```python
from build123d import *

# Parameters (mm, degrees)
F0_R         = 1.6
F1_DEPTH     = 5
F2_DEPTH     = 1
F3_R         = 16
F3_R_2       = 14.5
F4_DEPTH     = 10
F5_SIZE2     = 1.5
F5_SIZE      = 1
F8_T4_ANGLE  = 185.4300536725
F8_S5_R      = 22.5
F8_T6_DEPTH  = 9
F8_T10_ANGLE = 185.4300536725
F8_S11_R     = 22.5
F8_T12_DEPTH = 9
F9_R         = 5
F10_DEPTH    = 3
F11_R        = 3.25
F12_DEPTH    = 5


# Not quite as in the source:
# - a fillet or chamfer that OpenCascade refuses, or shapes differently, is made with other operations: its cross-section is extruded or revolved along the edge and cut away or added
# - a feature of the source that left no trace in its solid (it failed there, or was rolled back) is left out


with BuildPart() as f1:
    # F0 (on Top) → F1 (new body)
    with BuildSketch(Plane.XY):
        with BuildLine():
            ThreePointArc((-22.1862745098, -3.7442253372), (-22.5, 0), (-22.1862745098, 3.7442253372))
            ThreePointArc((-22.1862745098, 3.7442253372), (-30.5, 0), (-22.1862745098, -3.7442253372))
        make_face()
        with Locations((-25.5, 0)):
            Circle(F0_R, mode=Mode.SUBTRACT)
        with BuildLine():
            ThreePointArc((-20.5, 0), (-20.9410183456, 2.0532136456), (-22.1862745098, 3.7442253372))
            ThreePointArc((-22.1862745098, 3.7442253372), (-22.5, 0), (-22.1862745098, -3.7442253372))
            ThreePointArc((-22.1862745098, -3.7442253372), (-20.9410183456, -2.0532136456), (-20.5, 0))
        make_face()
    extrude(amount=F1_DEPTH)



with BuildPart() as f1b:
    # F0 (on Top) → F1, piece 2 (new body)
    with BuildSketch(Plane.XY):
        with BuildLine():
            ThreePointArc((22.1862745098, 3.7442253372), (22.4214314493, 1.8786728733), (22.5, 0))
            ThreePointArc((22.5, 0), (22.4214314493, -1.8786728733), (22.1862745098, -3.7442253372))
            ThreePointArc((22.1862745098, -3.7442253372), (27.5532136456, -4.5589816544), (30.5, 0))
            ThreePointArc((30.5, 0), (27.5532136456, 4.5589816544), (22.1862745098, 3.7442253372))
        make_face()
        with Locations((25.5, 0)):
            Circle(F0_R, mode=Mode.SUBTRACT)
        with BuildLine():
            ThreePointArc((22.1862745098, -3.7442253372), (22.4214314493, -1.8786728733), (22.5, 0))
            ThreePointArc((22.5, 0), (22.4214314493, 1.8786728733), (22.1862745098, 3.7442253372))
            ThreePointArc((22.1862745098, 3.7442253372), (20.5, 0), (22.1862745098, -3.7442253372))
        make_face()
    extrude(amount=F1_DEPTH)


with BuildPart() as f1_1:
    add(f1.part)

    add(f1b.part)  # F2 merges F1b
    # F0 (on Top) → F2 (join)
    with BuildSketch(Plane.XY):
        with BuildLine():
            ThreePointArc((22.1862745098, -3.7442253372), (20.5, 0), (22.1862745098, 3.7442253372))
            ThreePointArc((22.1862745098, 3.7442253372), (0, 22.5), (-22.1862745098, 3.7442253372))
            ThreePointArc((-22.1862745098, 3.7442253372), (-20.9410183456, 2.0532136456), (-20.5, 0))
            ThreePointArc((-20.5, 0), (-20.9410183456, -2.0532136456), (-22.1862745098, -3.7442253372))
            ThreePointArc((-22.1862745098, -3.7442253372), (0, -22.5), (22.1862745098, -3.7442253372))
        make_face()
    extrude(amount=F2_DEPTH)

    # F3 (on face) → F4 (join)
    with BuildSketch(Plane.XY.offset(1)):
        Circle(F3_R)
        Circle(F3_R_2, mode=Mode.SUBTRACT)
    extrude(amount=F4_DEPTH)

    # F5
    f5_edges = [f1_1.edges().sort_by_distance(p)[0] for p in [
        (-16, 0, 11),
    ]]
    f5_side = f1_1.faces().sort_by_distance((-15.547452, 0, 11))[0]
    chamfer(f5_edges, length=F5_SIZE, length2=F5_SIZE2, reference=f5_side)

    # F8: chamfer of 1.5 on 2 edges, made by hand


with BuildPart() as f8_tool2:
    # F8_s3 → F8_t4 (revolve)
    with BuildSketch(Plane(origin=(25.4427839223, 1.2065389767, 0), x_dir=(0, 0, 1), z_dir=(0.9988774861, 0.0473684257, 0))):
        Polygon((1, 7.7078948555), (2.5, 6.2078948555), (1, 6.2078948555), align=None)
    revolve(axis=Axis((25.5, 0, 1), (0, 0, -1)), revolution_arc=F8_T4_ANGLE)

    # F8_s5 → F8_t6 (intersect, symmetric)
    with BuildSketch(Plane.XY.offset(1.8)):
        Circle(F8_S5_R)
    extrude(amount=F8_T6_DEPTH, both=True, mode=Mode.INTERSECT)


with BuildPart() as f1_2:
    add(f1_1.part)

    # F8_t1: union F8_tool2
    add(f8_tool2.part)


with BuildPart() as f8_tool8:
    # F8_s9 → F8_t10 (revolve)
    with BuildSketch(Plane(origin=(-25.4427839223, 1.2065389767, 0), x_dir=(0, 0, 1), z_dir=(-0.9988774861, 0.0473684257, 0))):
        Polygon((1, -7.7078948555), (2.5, -6.2078948555), (1, -6.2078948555), align=None)
    revolve(axis=Axis((-25.5, 0, 1), (0, 0, 1)), revolution_arc=F8_T10_ANGLE)

    # F8_s11 → F8_t12 (intersect, symmetric)
    with BuildSketch(Plane.XY.offset(1.7)):
        Circle(F8_S11_R)
    extrude(amount=F8_T12_DEPTH, both=True, mode=Mode.INTERSECT)


with BuildPart() as f1_3:
    add(f1_2.part)

    # F8_t7: union F8_tool8
    add(f8_tool8.part)

    # F9 (on face) → F10 (join)
    with BuildSketch(Plane.XY.offset(1)):
        Circle(F9_R)
    extrude(amount=F10_DEPTH)

    # F11 (on face) → F12 (cut)
    with BuildSketch(Plane.XY.offset(4)):
        Circle(F11_R)
    extrude(amount=-F12_DEPTH, mode=Mode.SUBTRACT)


solid = f1_3.part
```
Source: CAD feature listing. Evaluate the final solid. Frame: model axes, mm. A direction names the side the tool comes from. Coordinates: 2 decimals unless noted, no trailing zeros. Loops run counter-clockwise (first coordinate to the right, second up) from the corner with the lowest first, then second, coordinate; pieces in that order, holes last. Notation, with made-up numbers: M 54,34 L 95,34 A15 cw 95,56 Z; hole C 35.5,-4 d11. An arc over 180 degrees is marked long. Use a Markdown table: item, result. Add a question column.
Q1. Section query C-C, the plane z = 6.5. Return loops of the section in (x, y).
Q2. Section query D-D, the plane x = -18. Return loops of the section in (y, z), and give its area (3 significant figures).
Q3. Draft query along Y for faces 1 (the cylindrical face through (-1.08, -4.88, 2.48)), 2 (the cylindrical face through (6.691, -12.864, 5.93)), 3 (the flat face through (24, 1, 5)), 4 (the conical face through (-20, 0, 2)). Return one class per face: pulls with the +Y half, pulls with the -Y half, needs draft (parallel to the pull), parting line crosses it, or undercut.
Q4. Material intervals for L1, parallel to Y at x = 0, z = 2.4; L2, parallel to Y at x = 25.5, z = 1.85; L3, parallel to Z at x = -18.5, y = 10, sorted ascending.
Q5. Section query B-B, the plane x = 0. Return loops of the section in (y, z), and give its area (3 significant figures).
Q6. First-contact query: pin 1 (3.5 mm diameter, centred on x = 25.5, y = 0, fed in from -Z); pin 2 (5 mm diameter, centred on x = -3.5, z = 7, fed in from -Y); pin 3 (8 mm diameter, centred on x = -17, y = -15, fed in from +Z); pin 4 (8 mm diameter, centred on x = 24, y = 0, fed in from +Z). Flat tips, straight axial feed; report the tip coordinate or a pass-through.
Q7. Section query A-A, the plane x = 25.5. Return loops of the section in (y, z).
Q8. Access query for faces 5 (the cylindrical face through (24.32, 1.08, 2.46)), 6 (the flat face through (-27, 1, 5)), 7 (the flat face through (6, 0, 1)). Directions: +Z, -Z, +X, -X, +Y, -Y. A direction counts if a zero-diameter tool reaches every point of the face in a straight line with its end or side. Return the directions, or none.
Result:
| question | item | result |
|---|---|---|
| 1 | outline | C 0,0 d32; hole C 0,0 d29 |
| 2 | outline | M -13.5,0 L 13.5,0 L 13.5,1 L -13.5,1 Z |
| 2 | area | 27.0 mm2 |
| 3 | face 1 | undercut |
| 3 | face 2 | undercut |
| 3 | face 3 | needs draft |
| 3 | face 4 | parting line crosses it |
| 4 | L1 | y = -16 to -14.5, -5 to -3.25, 3.25 to 5, 14.5 to 16 |
| 4 | L2 | y = -5 to -1.6, 1.6 to 5 |
| 4 | L3 | z = 0 to 1 |
| 5 | outline | M -22.5,0 L -3.25,0 L -3.25,4 L -5,4 L -5,1 L -14.5,1 L -14.5,11 L -15,11 L -16,9.5 L -16,1 L -22.5,1 Z; M 3.25,0 L 22.5,0 L 22.5,1 L 16,1 L 16,9.5 L 15,11 L 14.5,11 L 14.5,1 L 5,1 L 5,4 L 3.25,4 Z |
| 5 | area | 77.5 mm2 |
| 6 | pin 1 | stops at z = 0 |
| 6 | pin 2 | stops at y = -15.97 |
| 6 | pin 3 | stops at z = 1 |
| 6 | pin 4 | stops at z = 5 |
| 7 | outline | M -5,0 L -1.6,0 L -1.6,5 L -5,5 Z; M 1.6,0 L 5,0 L 5,5 L 1.6,5 Z |
| 8 | face 5 | +Z, -Z |
| 8 | face 6 | +Z, -X, +Y, -Y |
| 8 | face 7 | +Z |
